Autodesk Inventor part; units mm, degrees
ref_plane "Work Plane1" through (-20.5, -15, 1) normal (0, 0, 1) x (1, 0, 0)
ref_plane "YZ Plane" through (0, 0, 0) normal (1, 0, 0) x (0, 1, 0)
ref_plane "XZ Plane" through (0, 0, 0) normal (0, 1, 0) x (-1, 0, 0)
sketch "Sketch1" plane through (0, 0, 0) normal (0, 0, 1) x (1, 0, 0)
  line L0 (10, -15) -> (-10, -15)
  line L1 (10, 15) -> (10, -15)
  line L2 (-10, 15) -> (10, 15)
  line L3 (-10, -15) -> (-10, 15)
  line L4 (9.6, -14.6) -> (-9.6, -14.6)
  line L5 (-9.6, -14.6) -> (-9.6, 14.6)
  line L6 (-9.6, 14.6) -> (9.6, 14.6)
  line L7 (9.6, 14.6) -> (9.6, -14.6)
  point P0 (0, 0)
  dimension "d0" = 0.4
ref_plane "Work Plane1" through (-20.5, -15, 1) normal (0, 0, 1) x (1, 0, 0)
extrude "Extrusion1" add sketch "Sketch1" along normal up to surface (1 mm away) contours L4 L5 L6 L7
sketch "Sketch2" plane through (-9.6, -14.6, 1) normal (0, 0, 1) x (1, 0, 0)
  circle A0 centre (-6.4, 18.6) radius 2
  circle A1 centre (25.6, 18.6) radius 2
  line L0 (0, 0) -> (0, 29.2)
  line L1 (19.2, 0) -> (0, 0)
  line L2 (19.2, 29.2) -> (19.2, 0)
  line L3 (0, 29.2) -> (19.2, 29.2)
  line L4 (-0.4, -4.9) -> (-0.4, 26.1) construction
  line L5 (23.6, -4.9) -> (23.6, 26.1) construction
  line L6 (28.6, 32) -> (-5.4, 32)
  line L7 (-5.4, 32) -> (-5.4, -4)
  line L8 (-5.4, -4) -> (28.6, -4)
  line L9 (28.6, -4) -> (28.6, 32)
  circle A2 centre (25.6, 18.6) radius 5
  circle A3 centre (-6.4, 18.6) radius 5
  point P0 (-5.4, 23.499)
  point P1 (-5.4, 13.701)
  point P2 (28.6, 14.6)
  point P3 (28.6, 22.6)
  dimension "d12" = 34
  dimension "d13" = 4
  dimension "d14" = 24
  dimension "d15" = 5
  dimension "d16" = 36
  dimension "d17" = 3
  dimension "d18" = 3
extrude "Extrusion2" add sketch "Sketch2" along normal blind 17 contours L7 L6 L9 A2 L8 A3 | L0 L3 L2 L1
sketch "Sketch4" plane through (-15, 17.4, 1) normal (0, 1, 0) x (1, 0, 0)
  circle A0 centre (17, -18) radius 12
  circle A1 centre (17, -18) radius 13.5
  line L0 (34, -17) -> (26, -17)
  point P0 (15, 1)
  dimension "d19" = 1.5
extrude "Extrusion3" cut sketch "Sketch4" against normal up to surface (36 mm away) contours A0 | A1
ref_plane "Work Plane2" through (0, -91, 1) normal (0, 0, 1) x (1, 0, 0)
ref_plane "Work Plane3" through (0, -91, 1) normal (0, 0, 1) x (1, 0, 0)
sketch "Sketch5" plane through (0, -91, 1) normal (0, 0, 1) x (1, 0, 0)
  circle A0 centre (-16, 95) radius 2
  circle A1 centre (16, 95) radius 2
  line L0 (19, 99) -> (19, 108.4)
  line L1 (19, 102) -> (-19.6499, 102)
  line L2 (-19.6499, 102) -> (-19.6499, 88)
  line L3 (-19.6499, 88) -> (19, 88)
  line L4 (19, 88) -> (19, 102)
  point P0 (0, 91)
  dimension "d22" = 14
  dimension "d23" = 7
  dimension "d24" = 3.6498
extrude "Extrusion4" add sketch "Sketch5" along normal blind 1
sketch "Sketch6" plane through (-9.6, -14.6, 1) normal (0, 0, -1) x (-1, 0, 0)
  line L0 (-30.1, -0.4) -> (10.9, -0.4)
  line L1 (-28.6, -4) -> (-28.6, 32)
  line L2 (5.4, 11.6) -> (5.4, -4)
  line L3 (-28.6, 0.521) -> (5.4, 0.521)
  line L4 (5.4, 0.521) -> (5.4, -4)
  line L5 (5.4, -4) -> (-28.6, -4)
  line L6 (-28.6, -4) -> (-28.6, 0.521)
  point P0 (-9.6, 14.6)
  point P1 (-28.6, -4)
  point P2 (5.4, 0.521)
extrude "Extrusion5" cut sketch "Sketch6" against normal mid plane 4
equation "\"d15\" = -0.5 * d14 + 0.5 * d12"
equation "\"d23\" = 0.5 * d22"
properties part number "MotorBracket"
Check sheet for the modelled part. Datum: model origin and axes. Units: mm. A direction names the side the tool comes from. Give positions to 0.01 mm unless a question says otherwise; leave off trailing zeros. Write each loop counter-clockwise with the first axis right and the second up, starting at its lowest first coordinate (ties: lowest second). Pieces come first, ordered by that corner, then holes. Notation, with made-up numbers: (-21.75, 7.25) - (3.25, 7.25) arc R8 ccw to (3.25, 11.25) - close; hole circle Ø3 at (26.5, -9.5). An arc over 180 degrees is marked (long way). Answer as a JSON object with one key per item and string values. Group by question number.
1) Sectioned sample at B-B (z = 4.25). Record the cut outline in (x, y), then the cut area to 3 significant figures.
2) Depth check by flat-ended pin: P1, Ø2.5, axis at y = 11, z = 9.5, coming from the -X side; P2, Ø2.5, axis at x = -17, y = 1, coming from the +Z side; P3, Ø0.8, axis at x = -18, z = 1.5, coming from the +Y side; P4, Ø2.5, axis at x = -16, y = 4, coming from the +Z side. Enter the tip coordinate at first touch or a pass-through.
3) Access from +Z, -Z, +X, -X, +Y, -Y to the whole of each face (thin tool, end or side, straight path). Record for faces 1 (the face through (9.6, 0.5, 0.5)), 2 (the face through (-17.4, -3, 1.5)), 3 (the face through (2, -16, 3)), 4 (the face through (-0.1, 14.6, 0.5)), 5 (the face through (-17.3, 11, 1.5)).
4) Sectioned sample at D-D (y = 14). Record the cut outline in (x, z).
5) Sectioned sample at A-A (x = -16). Record the cut outline in (y, z), then the cut area to 3 significant figures.
6) Release check for a two-part mould opening along Y. For faces 6 (the face through (14.4, 5.2, 1.5)), 7 (the face through (2, -18.6, 5)), 8 (the face through (17, -9, 18)) record: pulls with the +Y half, pulls with the -Y half, needs draft (parallel to the pull), parting line crosses it, or undercut.
7) Sectioned sample at C-C (y = 4). Record the cut outline in (x, z).
8) Thickness scan on probe 1 along X at (y, z) = (3, 1.5); probe 2 along Y at (x, z) = (16, 1.3); probe 3 along Y at (x, z) = (16, 14). Record the ranges inside material, lowest first. Write a range as from..to.
Geometry results:
{
 "1": {"outline": "(-15, -18.6) - (19, -18.6) - (19, 0) arc R5 cw (long way) to (19, 8) - (19, 17.4) - (-15, 17.4) - (-15, 8.9) arc R5 cw to (-15, -0.9) - close", "area": "1,130 mm^2"},
 "2": {"P1": "stops at x = -15", "P2": "stops at z = 2", "P3": "stops at y = 11", "P4": "passes through"},
 "3": {"face 1": "-Z, +X, +Y, -Y", "face 2": "+Z, -Z, -X, -Y", "face 3": "-Z, +X, -X, -Y", "face 4": "-Z, +X, -X, +Y", "face 5": "+Z, -Z, -X, +Y"},
 "4": {"outline": "(-15, 1) - (-9.6, 1) - (-9.6, 0) - (9.6, 0) - (9.6, 1) - (19, 1) - (19, 18) - (15.46, 18) arc R13.5 cw to (-11.46, 18) - (-15, 18) - close"},
 "5": {"outline": "(-3, 1) - (2, 1) - (2, 2) - (-3, 2) - close; (6, 1) - (11, 1) - (11, 2) - (6, 2) - close", "area": "10.0 mm^2"},
 "6": {"face 6": "undercut", "face 7": "pulls with the -Y half", "face 8": "needs draft"},
 "7": {"outline": "(-19.65, 1) - (-18, 1) - (-18, 2) - (-19.65, 2) - close; (-14, 1) - (-9.6, 1) - (-9.6, 0) - (9.6, 0) - (9.6, 1) - (14, 1) - (14, 2) - (11, 2) - (11, 8.94) arc R13.5 cw to (-11, 15.36) - (-11, 2) - (-14, 2) - close; (18, 1) - (19, 1) - (19, 2) - (18, 2) - close"},
 "8": {"probe 1": "x = -19.65..-17.73, -14.27..14.27, 17.73..19", "probe 2": "y = -14.08..2, 6..17.4", "probe 3": "y = -18.6..-1, 9..17.4"}
}
